Part model, mm, in its own coordinate system. Face numbers are marked on the shaded views. A direction names the side the tool comes from. Round coordinates to 2 decimals unless told otherwise and drop trailing zeros. Write each loop counter-clockwise with the first axis right and the second up, starting at its lowest first coordinate (ties: lowest second). Pieces come first, ordered by that corner, then holes. Notation, with made-up numbers: M 64.25,-11.75 L 84.25,-11.75 A23 cw 84.25,-1.75 Z; hole C 43,44 d2. An arc over 180 degrees is marked long. Use one line per item in the form item = value. Start each with the question number.
Item 1: Probe L1, parallel to Y at x = 0, z = 5.5; L2, parallel to Y at x = -4.5, z = 4.75; L3, parallel to Y at x = 4, z = 5.5. List the from-to ranges inside material, lowest first.
Item 2: Cut at D-D, the plane y = 9. Give the cut face in (x, z).
Item 3: Cut at C-C, the plane z = 1.25. Give the cut face in (x, y).
Item 4: Mould opens along X. For the marked faces 3, 4 and 5 say: +X half, -X half, draft (parallel to the pull), parting line (faces both ways), or undercut.
Item 5: Cut at B-B, the plane x = 15. Give the cut face in (y, z), then the cut area to 3 significant figures.
Item 6: Which spindle directions (+Z, -Z, +X, -X, +Y, -Y) get a long thin tool onto all of the face, cutting with end or side? Do the marked faces 1 and 2. Say none if no direction does.
Item 7: Flat gauge pins, fed straight in: pin 1 Ø1 at (y, z) = (-6, 9.5) entering from -X; pin 2 Ø5.5 at (x, y) = (0, 0) entering from -Z; pin 3 Ø4 at (y, z) = (-10, 5) entering from -X; pin 4 Ø1.5 at (y, z) = (1.5, 4.5) entering from -X. Where does each tip first touch, or does it go through?
Item 8: Cut at A-A, the plane z = 8.25. Give the cut face in (x, y), then the cut area to 3 significant figures.
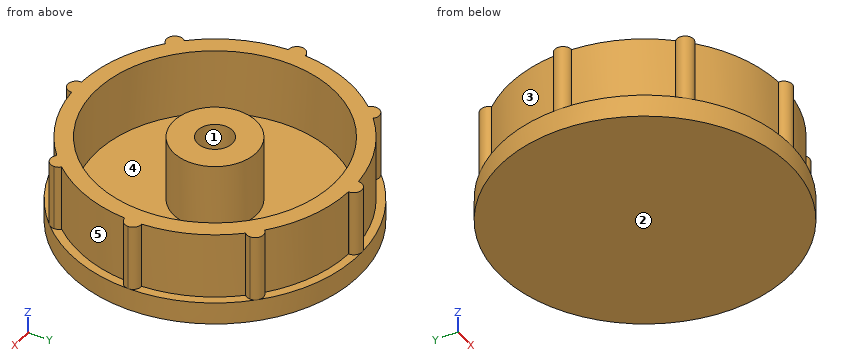
from build123d import *

# Parameters (mm, degrees)
F0_R     = 17.45
F1_DEPTH = 2.7
F2_R     = 14.45
F3_DEPTH = 8
F4_R     = 5
F4_R_2   = 2.1
F5_DEPTH = 8


with BuildPart() as f1:
    # F0 (on Top) → F1 (new body)
    with BuildSketch(Plane.XY):
        Circle(F0_R)
    extrude(amount=F1_DEPTH)

    # F2 (on face) → F3 (join)
    with BuildSketch(Plane.XY.offset(2.7)):
        with BuildLine():
            ThreePointArc((16.4196048632, -0.9995379611), (16.4423994599, -0.5), (16.45, 0))
            ThreePointArc((16.45, 0), (16.4423994599, 0.5), (16.4196048632, 0.9995379611))
            ThreePointArc((16.4196048632, 0.9995379611), (15.45, 0), (16.4196048632, -0.9995379611))
        make_face()
        with BuildLine():
            ThreePointArc((16.4196048632, 0.9995379611), (16.4423994599, 0.5), (16.45, 0))
            ThreePointArc((16.45, 0), (16.4423994599, -0.5), (16.4196048632, -0.9995379611))
            ThreePointArc((16.4196048632, -0.9995379611), (17.1462775536, -0.7177726439), (17.45, 0))
            ThreePointArc((17.45, 0), (17.1462775536, 0.7177726439), (16.4196048632, 0.9995379611))
        make_face()
        with BuildLine():
            ThreePointArc((16.4196048632, -0.9995379611), (15.45, 0), (16.4196048632, 0.9995379611))
            ThreePointArc((16.4196048632, 0.9995379611), (15.1978183098, 6.2951424624), (12.3171940135, 10.9036338728))
            ThreePointArc((12.3171940135, 10.9036338728), (10.9247997693, 10.9247997693), (10.9036338728, 12.3171940135))
            ThreePointArc((10.9036338728, 12.3171940135), (6.2951424624, 15.1978183098), (0.9995379611, 16.4196048632))
            ThreePointArc((0.9995379611, 16.4196048632), (0, 15.45), (-0.9995379611, 16.4196048632))
            ThreePointArc((-0.9995379611, 16.4196048632), (-6.2951424624, 15.1978183098), (-10.9036338728, 12.3171940135))
            ThreePointArc((-10.9036338728, 12.3171940135), (-10.7023172117, 12.0005034322), (-10.6319065505, 11.6319065505))
            ThreePointArc((-10.6319065505, 11.6319065505), (-11.2352249799, 10.7139502708), (-12.3171940135, 10.9036338728))
            ThreePointArc((-12.3171940135, 10.9036338728), (-15.1978183098, 6.2951424624), (-16.4196048632, 0.9995379611))
            ThreePointArc((-16.4196048632, 0.9995379611), (-15.7322273561, 0.6962775536), (-15.45, 0))
            ThreePointArc((-15.45, 0), (-15.7322273561, -0.6962775536), (-16.4196048632, -0.9995379611))
            ThreePointArc((-16.4196048632, -0.9995379611), (-15.1978183098, -6.2951424624), (-12.3171940135, -10.9036338728))
            ThreePointArc((-12.3171940135, -10.9036338728), (-11.2352249799, -10.7139502708), (-10.6319065505, -11.6319065505))
            ThreePointArc((-10.6319065505, -11.6319065505), (-10.7023172117, -12.0005034322), (-10.9036338728, -12.3171940135))
            ThreePointArc((-10.9036338728, -12.3171940135), (-6.2951424624, -15.1978183098), (-0.9995379611, -16.4196048632))
            ThreePointArc((-0.9995379611, -16.4196048632), (0, -15.45), (0.9995379611, -16.4196048632))
            ThreePointArc((0.9995379611, -16.4196048632), (6.2951424624, -15.1978183098), (10.9036338728, -12.3171940135))
            ThreePointArc((10.9036338728, -12.3171940135), (10.9247997693, -10.9247997693), (12.3171940135, -10.9036338728))
            ThreePointArc((12.3171940135, -10.9036338728), (15.1978183098, -6.2951424624), (16.4196048632, -0.9995379611))
        make_face()
        Circle(F2_R, mode=Mode.SUBTRACT)
        with BuildLine():
            ThreePointArc((10.9036338728, 12.3171940135), (10.9247997693, 10.9247997693), (12.3171940135, 10.9036338728))
            ThreePointArc((12.3171940135, 10.9036338728), (11.6319065505, 11.6319065505), (10.9036338728, 12.3171940135))
        make_face()
        with BuildLine():
            ThreePointArc((10.9036338728, 12.3171940135), (11.6319065505, 11.6319065505), (12.3171940135, 10.9036338728))
            ThreePointArc((12.3171940135, 10.9036338728), (12.5498628303, 11.2352249799), (12.6319065505, 11.6319065505))
            ThreePointArc((12.6319065505, 11.6319065505), (12.0005034322, 12.5614958893), (10.9036338728, 12.3171940135))
        make_face()
        with BuildLine():
            ThreePointArc((12.6319065505, -11.6319065505), (12.5498628303, -11.2352249799), (12.3171940135, -10.9036338728))
            ThreePointArc((12.3171940135, -10.9036338728), (11.6319065505, -11.6319065505), (10.9036338728, -12.3171940135))
            ThreePointArc((10.9036338728, -12.3171940135), (12.0005034322, -12.5614958893), (12.6319065505, -11.6319065505))
        make_face()
        with BuildLine():
            ThreePointArc((10.9036338728, -12.3171940135), (11.6319065505, -11.6319065505), (12.3171940135, -10.9036338728))
            ThreePointArc((12.3171940135, -10.9036338728), (10.9247997693, -10.9247997693), (10.9036338728, -12.3171940135))
        make_face()
        with BuildLine():
            ThreePointArc((-0.9995379611, 16.4196048632), (0, 15.45), (0.9995379611, 16.4196048632))
            ThreePointArc((0.9995379611, 16.4196048632), (0, 16.45), (-0.9995379611, 16.4196048632))
        make_face()
        with BuildLine():
            ThreePointArc((-0.9995379611, 16.4196048632), (0, 16.45), (0.9995379611, 16.4196048632))
            ThreePointArc((0.9995379611, 16.4196048632), (0.9998844836, 16.4348006758), (1, 16.45))
            ThreePointArc((1, 16.45), (-0.0151993242, 17.4498844836), (-0.9995379611, 16.4196048632))
        make_face()
        with BuildLine():
            ThreePointArc((1, -16.45), (0.9998844836, -16.4348006758), (0.9995379611, -16.4196048632))
            ThreePointArc((0.9995379611, -16.4196048632), (0, -16.45), (-0.9995379611, -16.4196048632))
            ThreePointArc((-0.9995379611, -16.4196048632), (-0.0151993242, -17.4498844836), (1, -16.45))
        make_face()
        with BuildLine():
            ThreePointArc((-0.9995379611, -16.4196048632), (0, -16.45), (0.9995379611, -16.4196048632))
            ThreePointArc((0.9995379611, -16.4196048632), (0, -15.45), (-0.9995379611, -16.4196048632))
        make_face()
        with BuildLine():
            ThreePointArc((-10.6319065505, 11.6319065505), (-10.7023172117, 12.0005034322), (-10.9036338728, 12.3171940135))
            ThreePointArc((-10.9036338728, 12.3171940135), (-11.6319065505, 11.6319065505), (-12.3171940135, 10.9036338728))
            ThreePointArc((-12.3171940135, 10.9036338728), (-11.2352249799, 10.7139502708), (-10.6319065505, 11.6319065505))
        make_face()
        with BuildLine():
            ThreePointArc((-12.3171940135, 10.9036338728), (-11.6319065505, 11.6319065505), (-10.9036338728, 12.3171940135))
            ThreePointArc((-10.9036338728, 12.3171940135), (-12.3390133317, 12.3390133317), (-12.3171940135, 10.9036338728))
        make_face()
        with BuildLine():
            ThreePointArc((-12.3171940135, -10.9036338728), (-12.3390133317, -12.3390133317), (-10.9036338728, -12.3171940135))
            ThreePointArc((-10.9036338728, -12.3171940135), (-11.6319065505, -11.6319065505), (-12.3171940135, -10.9036338728))
        make_face()
        with BuildLine():
            ThreePointArc((-12.3171940135, -10.9036338728), (-11.6319065505, -11.6319065505), (-10.9036338728, -12.3171940135))
            ThreePointArc((-10.9036338728, -12.3171940135), (-10.7023172117, -12.0005034322), (-10.6319065505, -11.6319065505))
            ThreePointArc((-10.6319065505, -11.6319065505), (-11.2352249799, -10.7139502708), (-12.3171940135, -10.9036338728))
        make_face()
        with BuildLine():
            ThreePointArc((-15.45, 0), (-15.7322273561, 0.6962775536), (-16.4196048632, 0.9995379611))
            ThreePointArc((-16.4196048632, 0.9995379611), (-16.45, 0), (-16.4196048632, -0.9995379611))
            ThreePointArc((-16.4196048632, -0.9995379611), (-15.7322273561, -0.6962775536), (-15.45, 0))
        make_face()
        with BuildLine():
            ThreePointArc((-16.4196048632, -0.9995379611), (-16.45, 0), (-16.4196048632, 0.9995379611))
            ThreePointArc((-16.4196048632, 0.9995379611), (-17.45, 0), (-16.4196048632, -0.9995379611))
        make_face()
    extrude(amount=F3_DEPTH)

    # F4 (on face) → F5 (join)
    with BuildSketch(Plane.XY.offset(2.7)):
        Circle(F4_R)
        Circle(F4_R_2, mode=Mode.SUBTRACT)
    extrude(amount=F5_DEPTH)


solid = f1.part
Model answer:
q1.L1 = -17.45 to -14.45, -5 to -2.1, 2.1 to 5, 14.45 to 17.45
q1.L2 = -15.82 to -13.73, -2.18 to 2.18, 13.73 to 15.82
q1.L3 = -15.96 to -13.89, -3 to 3, 13.89 to 15.96
q2.outline = M -14.95,0 L 14.95,0 L 14.95,2.7 L 13.77,2.7 L 13.77,10.7 L 11.3,10.7 L 11.3,2.7 L -11.3,2.7 L -11.3,10.7 L -13.77,10.7 L -13.77,2.7 L -14.95,2.7 Z
q3.outline = C 0,0 d34.9
q4.face_3 = -X half
q4.face_4 = undercut
q4.face_5 = +X half
q5.outline = M -8.92,0 L 8.92,0 L 8.92,2.7 L 6.75,2.7 L 6.75,10.7 L -6.75,10.7 L -6.75,2.7 L -8.92,2.7 Z
q5.area = 156 mm²
q6.face_1 = +Z
q6.face_2 = -Z, +X, -X, +Y, -Y
q7.pin_1 = -15.5
q7.pin_2 = 0
q7.pin_3 = -14.37
q7.pin_4 = -17.11
q8.outline = M -16.42,-1 A16.45 ccw -12.32,-10.9 A1 ccw long -10.9,-12.32 A16.45 ccw -1,-16.42 A1 ccw long 1,-16.42 A16.45 ccw 10.9,-12.32 A1 ccw long 12.32,-10.9 A16.45 ccw 16.42,-1 A1 ccw long 16.42,1 A16.45 ccw 12.32,10.9 A1 ccw long 10.9,12.32 A16.45 ccw 1,16.42 A1 ccw long -1,16.42 A16.45 ccw -10.9,12.32 A1 ccw long -12.32,10.9 A16.45 ccw -16.42,1 A1 ccw long Z; C 0,0 d10; hole C 0,0 d28.9; hole C 0,0 d4.2
q8.area = 272 mm²
